from build123d import *

# Parameters (mm, degrees)
SKETCH1_W               = 94
SKETCH1_H               = 36
BOSS_EXTRUDE1_DEPTH     = 10
SKETCH2_W               = 36
SKETCH2_H               = 7
BOSS_EXTRUDE2_DEPTH     = 90
CUT_EXTRUDE1_DEPTH      = 139.419651784
CUT_EXTRUDE1_DEPTH_BACK = 139.419651784
SKETCH3_R               = 3.5
CUT_EXTRUDE2_DEPTH      = 139.419651784
CUT_EXTRUDE2_DEPTH_BACK = 3
SKETCH4_R               = 7
CUT_EXTRUDE3_START      = -3
SKETCH5_R               = 7
CUT_EXTRUDE3_DEPTH      = 3
FILLET1_R               = 18
SKETCH6_R               = 7.5
BOSS_EXTRUDE3_DEPTH     = 8
SKETCH7_R               = 4.5
CUT_EXTRUDE4_DEPTH      = 120.151164493
FILLET2_R               = 2
SKETCH9_R               = 0.75
SKETCH9_W               = 22.5
SKETCH9_H               = 11.8
CUT_EXTRUDE5_DEPTH      = 104.116439039
SKETCH10_W              = 33
SKETCH10_H              = 15
CUT_EXTRUDE6_DEPTH      = 4
SKETCH11_W              = 17
SKETCH11_H              = 32
BOSS_EXTRUDE4_DEPTH     = 7
CUT_EXTRUDE7_REACH      = 143.515
SKETCH12_R              = 0.75
SKETCH12_W              = 11.8
SKETCH12_H              = 22.5
CUT_EXTRUDE8_START      = -5
CUT_EXTRUDE8_DEPTH      = 5
FILLET3_R               = 1.5
FILLET4_R               = 4


# Some blends are built 0.0001 mm under size
with BuildPart() as part:
    # Sketch1 → Boss-Extrude1 (new body)
    with BuildSketch(Plane(origin=(0, 0, 0), x_dir=(0, 1, 0), z_dir=(0, 0, 1))):
        Rectangle(SKETCH1_W, SKETCH1_H)
    extrude(amount=BOSS_EXTRUDE1_DEPTH)

    # Sketch2 → Boss-Extrude2 (add)
    with BuildSketch(Plane.XY.offset(10)):
        with Locations((0, 43.5)):
            Rectangle(SKETCH2_W, SKETCH2_H)
        with Locations((0, -43.5)):
            Rectangle(SKETCH2_W, SKETCH2_H)
    extrude(amount=BOSS_EXTRUDE2_DEPTH)

    # Sketch3 → Cut-Extrude1 (cut, two sides: drawn at the far end of the back side and taken through both)
    with BuildSketch(Plane.XZ.offset(47).offset(-CUT_EXTRUDE1_DEPTH_BACK)):
        with Locations(Location((0, 82, 0), (0, 0, 270))):
            Circle(SKETCH3_R)
    extrude(amount=CUT_EXTRUDE1_DEPTH + CUT_EXTRUDE1_DEPTH_BACK, mode=Mode.SUBTRACT)

    # Sketch4 → Cut-Extrude2 (cut, two sides: drawn at the far end of the back side and taken through both)
    with BuildSketch(Plane.XZ.offset(47).offset(-CUT_EXTRUDE2_DEPTH_BACK)):
        with Locations(Location((0, 82, 0), (0, 0, 90))):
            Circle(SKETCH4_R)
    extrude(amount=CUT_EXTRUDE2_DEPTH + CUT_EXTRUDE2_DEPTH_BACK, mode=Mode.SUBTRACT)

    # Sketch5 → Cut-Extrude3 (cut)
    with BuildSketch(Plane(origin=(0, 47, 0), x_dir=(-1, 0, 0), z_dir=(0, 1, 0)).offset(CUT_EXTRUDE3_START)):
        with Locations(Location((0, 82, 0), (0, 0, 90))):
            Circle(SKETCH5_R)
    extrude(amount=CUT_EXTRUDE3_DEPTH, mode=Mode.SUBTRACT)

    # Fillet1
    fillet1_edges = [part.edges().sort_by_distance(p)[0] for p in [
        (18, -43.5, 100),
        (-18, -43.5, 100),
        (18, 43.5, 100),
        (-18, 43.5, 100),
    ]]
    fillet(fillet1_edges, radius=FILLET1_R - 0.0001)  # a hair under: the kernel refuses the full size

    # Sketch6 → Boss-Extrude3 (add)
    with BuildSketch(Plane(origin=(0, 0, 0), x_dir=(1, 0, 0), z_dir=(0, 0, -1))):
        with Locations(Location((0, 0, 0), (0, 0, 180))):
            Circle(SKETCH6_R)
    extrude(amount=BOSS_EXTRUDE3_DEPTH)

    # Sketch7 → Cut-Extrude4 (cut, through all)
    with BuildSketch(Plane(origin=(0, 0, -8), x_dir=(1, 0, 0), z_dir=(0, 0, -1))):
        with Locations(Location((0, 0, 0), (0, 0, 180))):
            Circle(SKETCH7_R)
    extrude(amount=-CUT_EXTRUDE4_DEPTH, mode=Mode.SUBTRACT)

    # Fillet2
    fillet2_edges = [part.edges().sort_by_distance(p)[0] for p in [
        (7.5, 0, 0),
    ]]
    fillet(fillet2_edges, radius=FILLET2_R)

    # Sketch9 → Cut-Extrude5 (cut, through all)
    with BuildSketch(Plane.XY.offset(10)):
        with Locations((-13.65, 27.484131785)):
            Circle(SKETCH9_R)
        with Locations((13.65, 27.484131785)):
            Circle(SKETCH9_R)
        with Locations((0, 27.484131785)):
            Rectangle(SKETCH9_W, SKETCH9_H)
    extrude(amount=-CUT_EXTRUDE5_DEPTH, mode=Mode.SUBTRACT)

    # Sketch10 → Cut-Extrude6 (cut)
    with BuildSketch(Plane.XY.offset(10)):
        with Locations((0, 27.484131785)):
            Rectangle(SKETCH10_W, SKETCH10_H)
    extrude(amount=-CUT_EXTRUDE6_DEPTH, mode=Mode.SUBTRACT)

    # Sketch11 → Boss-Extrude4 (add)
    with BuildSketch(Plane(origin=(0, 47, 0), x_dir=(-1, 0, 0), z_dir=(0, 1, 0))):
        with Locations((-26.003605519, 66)):
            Rectangle(SKETCH11_W, SKETCH11_H)
    extrude(amount=-BOSS_EXTRUDE4_DEPTH)

    # Sketch12 → Cut-Extrude7 (cut, up to next)
    with BuildSketch(Plane(origin=(0, 47, 0), x_dir=(-1, 0, 0), z_dir=(0, 1, 0)), mode=Mode.PRIVATE) as cut_extrude7_sk1:
        with Locations(Location((-26.003605519, 79.65, 0), (0, 0, 90))):
            Circle(SKETCH12_R)
    cut_extrude7_tool1 = extrude(cut_extrude7_sk1.sketch, amount=-CUT_EXTRUDE7_REACH, mode=Mode.PRIVATE) & part.part
    # Sketch12 → Cut-Extrude7 (cut, up to next)
    with BuildSketch(Plane(origin=(0, 47, 0), x_dir=(-1, 0, 0), z_dir=(0, 1, 0)), mode=Mode.PRIVATE) as cut_extrude7_sk2:
        with Locations((-26.003605519, 52.35)):
            Circle(SKETCH12_R)
    cut_extrude7_tool2 = extrude(cut_extrude7_sk2.sketch, amount=-CUT_EXTRUDE7_REACH, mode=Mode.PRIVATE) & part.part
    # Sketch12 → Cut-Extrude7 (cut, up to next)
    with BuildSketch(Plane(origin=(0, 47, 0), x_dir=(-1, 0, 0), z_dir=(0, 1, 0)), mode=Mode.PRIVATE) as cut_extrude7_sk3:
        with Locations((-26.003605519, 66)):
            Rectangle(SKETCH12_W, SKETCH12_H)
    cut_extrude7_tool3 = extrude(cut_extrude7_sk3.sketch, amount=-CUT_EXTRUDE7_REACH, mode=Mode.PRIVATE) & part.part
    add(cut_extrude7_tool1.solids().sort_by_distance((26.003606, 47, 79.65))[0], mode=Mode.SUBTRACT)
    add(cut_extrude7_tool2.solids().sort_by_distance((26.003606, 47, 52.35))[0], mode=Mode.SUBTRACT)
    add(cut_extrude7_tool3.solids().sort_by_distance((26.003606, 47, 66))[0], mode=Mode.SUBTRACT)

    # Sketch13 → Cut-Extrude8 (cut)
    with BuildSketch(Plane.XY.offset(10).offset(CUT_EXTRUDE8_START)):
        with BuildLine():
            Line((18, -7.5), (18, 7.5))
            Line((18, 7.5), (-0.72547331, 4.441135944))
            ThreePointArc((-0.72547331, 4.441135944), (4.5, 0), (-0.72547331, -4.441135944))
            Line((-0.72547331, -4.441135944), (18, -7.5))
        make_face()
    extrude(amount=CUT_EXTRUDE8_DEPTH, mode=Mode.SUBTRACT)

    # Fillet3
    fillet3_edges = [part.edges().sort_by_distance(p)[0] for p in [
        (-18, 0, 10),
        (18, -23.75, 10),
        (-3.428894129, 2.914221174, 10),
        (18, 23.75, 10),
        (8.637263345, -5.970567972, 10),
        (8.637263345, 5.970567972, 10),
    ]]
    fillet(fillet3_edges, radius=FILLET3_R - 0.0001)  # a hair under: the kernel refuses the full size

    # Fillet4
    # the kernel refuses this fillet: 4 mm, written as the material it adds along each edge
    with BuildSketch(Plane(origin=(16.5001, 40, 10), x_dir=(0, -1, 0), z_dir=(-1, 0, 0))) as fillet4_piece_1:
        with BuildLine():
            CenterArc((FILLET4_R, FILLET4_R), FILLET4_R, 180, 90)
            Line((0, FILLET4_R), (0, 0))
            Line((0, 0), (FILLET4_R, 0))
        make_face()
    extrude(amount=33.0002)
    with BuildSketch(Plane(origin=(16.5001, -40, 10), x_dir=(0, 1, 0), z_dir=(-1, 0, 0))) as fillet4_piece_2:
        with BuildLine():
            CenterArc((FILLET4_R, -FILLET4_R), FILLET4_R, 90, 90)
            Line((0, -FILLET4_R), (0, 0))
            Line((0, 0), (FILLET4_R, 0))
        make_face()
    extrude(amount=33.0002)
    with BuildSketch(Plane(origin=(-16.5001, -40, 8.5001), x_dir=(0.006283143965556653, 0, 0.9999802608561371), z_dir=(-0.9999802608561371, 0, 0.006283143965556653))) as fillet4_piece_3_section:
        with BuildLine():
            CenterArc((-1.4999 - FILLET4_R, FILLET4_R), FILLET4_R, 270, 90)
            Line((-1.4999 - FILLET4_R, 0), (-1.4999, 0))
            Line((-1.4999, 0), (-1.4999, FILLET4_R))
        make_face()
    fillet4_piece_3 = revolve(axis=Axis((-16.5001, -40, 8.5001), (0, 1, 0)), revolution_arc=359.64, mode=Mode.PRIVATE)
    fillet4_piece_3 = split(fillet4_piece_3, bisect_by=Plane(origin=(-18, -38.511467158, 9.644627934), z_dir=(1, 0, 0)), keep=Keep.TOP, mode=Mode.PRIVATE)
    add(fillet4_piece_3)
    with BuildSketch(Plane(origin=(-16.5001, 40, 8.5001), x_dir=(0.006283143965556653, 0, 0.9999802608561371), z_dir=(-0.9999802608561371, 0, 0.006283143965556653))) as fillet4_piece_4_section:
        with BuildLine():
            CenterArc((-1.4999 - FILLET4_R, -FILLET4_R), FILLET4_R, 0, 90)
            Line((-1.4999 - FILLET4_R, 0), (-1.4999, 0))
            Line((-1.4999, 0), (-1.4999, -FILLET4_R))
        make_face()
    fillet4_piece_4 = revolve(axis=Axis((-16.5001, 40, 8.5001), (0, 1, 0)), revolution_arc=359.64, mode=Mode.PRIVATE)
    fillet4_piece_4 = split(fillet4_piece_4, bisect_by=Plane(origin=(-18, 38.511467158, 9.644627939), z_dir=(1, 0, 0)), keep=Keep.TOP, mode=Mode.PRIVATE)
    add(fillet4_piece_4)
    with BuildSketch(Plane(origin=(16.5001, -40, 8.5001), x_dir=(-0.006283143965559021, 0, 0.9999802608561371), z_dir=(0.9999802608561371, 0, 0.006283143965559021))) as fillet4_piece_5_section:
        with BuildLine():
            CenterArc((-1.4999 - FILLET4_R, -FILLET4_R), FILLET4_R, 0, 90)
            Line((-1.4999 - FILLET4_R, 0), (-1.4999, 0))
            Line((-1.4999, 0), (-1.4999, -FILLET4_R))
        make_face()
    fillet4_piece_5 = revolve(axis=Axis((16.5001, -40, 8.5001), (0, -1, 0)), revolution_arc=359.64, mode=Mode.PRIVATE)
    fillet4_piece_5 = split(fillet4_piece_5, bisect_by=Plane(origin=(18, -38.511467161, 9.644627937), z_dir=(-1, 0, 0)), keep=Keep.TOP, mode=Mode.PRIVATE)
    add(fillet4_piece_5)
    with BuildSketch(Plane(origin=(16.5001, 40, 8.5001), x_dir=(-0.006283143965559021, 0, 0.9999802608561371), z_dir=(0.9999802608561371, 0, 0.006283143965559021))) as fillet4_piece_6_section:
        with BuildLine():
            CenterArc((-1.4999 - FILLET4_R, FILLET4_R), FILLET4_R, 270, 90)
            Line((-1.4999, FILLET4_R), (-1.4999, 0))
            Line((-1.4999, 0), (-1.4999 - FILLET4_R, 0))
        make_face()
    fillet4_piece_6 = revolve(axis=Axis((16.5001, 40, 8.5001), (0, -1, 0)), revolution_arc=359.64, mode=Mode.PRIVATE)
    fillet4_piece_6 = split(fillet4_piece_6, bisect_by=Plane(origin=(18, 38.511467202, 9.644627972), z_dir=(-1, 0, 0)), keep=Keep.TOP, mode=Mode.PRIVATE)
    add(fillet4_piece_6)
    # the kernel refuses this fillet: 4 mm, written as the material it takes off along each edge
    with BuildSketch(Plane(origin=(-28, -47, 0), x_dir=(0, 0, 1), z_dir=(1, 0, 0))) as fillet4_2_piece_1:
        with BuildLine():
            CenterArc((FILLET4_R, -FILLET4_R), FILLET4_R, 90, 90)
            Line((0, -FILLET4_R), (0, 0))
            Line((0, 0), (FILLET4_R, 0))
        make_face()
    extrude(amount=56, mode=Mode.SUBTRACT)
    with BuildSketch(Plane(origin=(28, 47, 0), x_dir=(0, -1, 0), z_dir=(-1, 0, 0))) as fillet4_2_piece_2:
        with BuildLine():
            CenterArc((FILLET4_R, FILLET4_R), FILLET4_R, 180, 90)
            Line((0, FILLET4_R), (0, 0))
            Line((0, 0), (FILLET4_R, 0))
        make_face()
    extrude(amount=56, mode=Mode.SUBTRACT)


solid = part.part
Part model, mm, in its own coordinate system. A direction names the side the tool comes from. Coordinates: 2 decimals unless noted, no trailing zeros. Loops run counter-clockwise (first coordinate to the right, second up) from the corner with the lowest first, then second, coordinate; pieces in that order, holes last. Notation, with made-up numbers: (-23.5, 38) -> (21.5, 38) arc R28 cw to (21.5, 63) -> close; hole circle Ø1 at (34.25, 3). An arc over 180 degrees is marked (long way). Use a Markdown table: item, result. Add a question column.
Item 1: Band-saw the part on C-C on z = 27. Write the cut outline in (x, y).
Item 2: Flat gauge pins, fed straight in: P1, Ø11, axis at x = 0, z = 82, coming from the +Y side; P2, Ø1.5, axis at x = 9.5, y = 3, coming from the +Z side; P3, Ø2, axis at x = -13.65, y = 27.48, coming from the -Z side. Where does each tip first touch, or does it go through?
Item 3: Band-saw the part on D-D on y = -23.5. Write the cut outline in (x, z), plus the area to 3 significant figures.
Item 4: Which spindle directions (+Z, -Z, +X, -X, +Y, -Y) get a long thin tool onto all of the face, cutting with end or side? Do faces 1 (the flat face through (0, 21.584, 3)), 2 (the flat face through (0, 34.984, 8)), 3 (the flat face through (26, 44, 54.75)). Say none if no direction does.
Item 5: Band-saw the part on B-B on y = 0. Write the cut outline in (x, z), plus the area to 3 significant figures.
Item 6: Pull direction Z, two halves, no side cores. Call faces 4 (the cylindrical face through (0, 45, 75)), 5 (the flat face through (11, 0, 5)), 6 (the flat face through (20.104, 44, 66)), 7 (the flat face through (0, 19.984, 8)): +Z half, -Z half, draft (parallel to the pull), parting line (faces both ways), or undercut.
Item 7: Probe probe 1 along Y at (x, z) = (-6.5, 53); probe 2 along X at (y, z) = (0, 0.25); probe 3 along X at (y, z) = (43.5, 79.65). List the from-to ranges inside material, lowest first.
Item 8: Band-saw the part on A-A on z = 61. Write the cut outline in (x, y), plus the area to 3 significant figures.
Geometry says:
| question | item | result |
|---|---|---|
| 1 | outline | (-18, -47) -> (18, -47) -> (18, -40) -> (-18, -40) -> close; (-18, 40) -> (18, 40) -> (18, 47) -> (-18, 47) -> close |
| 2 | P1 | y = 44 |
| 2 | P2 | z = 5 |
| 2 | P3 | z = 0 |
| 3 | outline | (-18, 0) -> (18, 0) -> (18, 8.5) arc R1.5 ccw to (16.5, 10) -> (-16.5, 10) arc R1.5 ccw to (-18, 8.5) -> close |
| 3 | area | 359 mm² |
| 4 | face 1 | +Z, -Z |
| 4 | face 2 | +Z |
| 4 | face 3 | +Y, -Y |
| 5 | outline | (-18, 0) -> (-9.5, 0) arc R2 cw to (-7.5, -2) -> (-7.5, -8) -> (-4.5, -8) -> (-4.5, 8.5) arc R1.5 ccw to (-6, 10) -> (-16.5, 10) arc R1.5 ccw to (-18, 8.5) -> close; (4.5, -8) -> (7.5, -8) -> (7.5, -2) arc R2 cw to (9.5, 0) -> (18, 0) -> (18, 5) -> (4.5, 5) -> close |
| 5 | area | 251 mm² |
| 6 | face 4 | undercut |
| 6 | face 5 | +Z half |
| 6 | face 6 | undercut |
| 6 | face 7 | draft |
| 7 | probe 1 | -47 to -40, 40 to 47 |
| 7 | probe 2 | -18 to -4.5, 4.5 to 18 |
| 7 | probe 3 | -18 to -2.59, 2.59 to 25.25, 26.75 to 34.5 |
| 8 | outline | (-18, -47) -> (18, -47) -> (18, -40) -> (-18, -40) -> close; (-18, 40) -> (20.1, 40) -> (20.1, 47) -> (-18, 47) -> close; (31.9, 40) -> (34.5, 40) -> (34.5, 47) -> (31.9, 47) -> close |
| 8 | area | 537 mm² |
